```python
from build123d import *

# Parameters (mm, degrees)
F0_W     = 25.4
F0_H     = 12.7
F0_W_2   = 12.7
F1_DEPTH = 12.7


with BuildPart() as f1:
    # F0 (on Front) → F1 (new body, symmetric)
    with BuildSketch(Plane.XZ):
        Polygon((0, 3.175), (0, 0), (76.2, 0), (76.2, 3.175), (76.2, 15.875), (76.2, 19.05), (0, 19.05), (0, 15.875), align=None)
        with Locations((-12.7, 9.525)):
            Rectangle(F0_W, F0_H)
        with Locations((82.55, 9.525)):
            Rectangle(F0_W_2, F0_H)
    extrude(amount=F1_DEPTH, both=True)


solid = f1.part
```
Design review of the part built by this model. Coordinates are the model's own, in mm. A direction names the side the tool comes from. Give positions to 0.01 mm unless a question says otherwise; leave off trailing zeros. Order: outer loops, then holes, each group sorted by start corner. A loop starts at its lowest first (then second) coordinate and runs counter-clockwise, first axis right, second up. Notation, with made-up numbers: M -7.5,-33.5 L 49.5,-33.5 A14 ccw 49.5,-13.5 Z; hole C -22,-27.5 d8. An arc over 180 degrees is marked long. One line per question, with ' | ' between items. Start each with the question number.
Q1. We need section B-B (x = 79.5). Write out the cut boundary in (y, z) (3 decimals).
Q2. We need section C-C (z = 17.25). Write out the cut boundary in (x, y), plus the area to 3 significant figures.
Q3. We need section A-A (y = 7.5). Write out the cut boundary in (x, z) (3 decimals).
Q4. For pin 1 Ø3 at (x, y) = (-4, 4) entering from -Z (3 decimals); pin 2 Ø1 at (y, z) = (4.5, 17) entering from +X; pin 3 Ø4 at (x, y) = (60.5, -6.5) entering from -Z; pin 4 Ø1 at (y, z) = (0, 17) entering from -X, all flat-tipped, find the tip position at first contact; note any pin that passes through.
Q5. For L1, parallel to X at y = 5.25, z = 2.5; L2, parallel to Z at x = -11, y = -4 (3 decimals), list the stretches that pass through material, from the lowest coordinate up. Write a range as [from, to].
Q6. Machinability: for faces 1 (the face through (-13, 0, 15.875)), 2 (the face through (0, 0, 2)), 3 (the face through (82, 0, 15.875)), which of the approach directions +Z, -Z, +X, -X, +Y, -Y give a long, thin tool a straight path to every point of the face, cutting with its end or side? Answer none if there is none.
Returned:
1) outline: M -12.7,3.175 L 12.7,3.175 L 12.7,15.875 L -12.7,15.875 Z
2) outline: M 0,-12.7 L 76.2,-12.7 L 76.2,12.7 L 0,12.7 Z | area: 1,940 mm2
3) outline: M -25.4,3.175 L 0,3.175 L 0,0 L 76.2,0 L 76.2,3.175 L 88.9,3.175 L 88.9,15.875 L 76.2,15.875 L 76.2,19.05 L 0,19.05 L 0,15.875 L -25.4,15.875 Z
4) pin 1: z = 3.175 | pin 2: x = 76.2 | pin 3: z = 0 | pin 4: x = 0
5) L1: [0, 76.2] | L2: [3.175, 15.875]
6) face 1: +Z, -X, +Y, -Y | face 2: -Z, -X, +Y, -Y | face 3: +Z, +X, +Y, -Y
